Design review of the part built by this model. Coordinates are the model's own, in mm. A direction names the side the tool comes from. Round coordinates to 2 decimals unless told otherwise and drop trailing zeros. Order: outer loops, then holes, each group sorted by start corner. A loop starts at its lowest first (then second) coordinate and runs counter-clockwise, first axis right, second up. Notation, with made-up numbers: (87.5, 78.25) - (132.5, 78.25) arc R22 cw to (132.5, 94.25) - close; hole circle Ø6 at (50.25, 4.25). An arc over 180 degrees is marked (long way). Use CSV: the item, a comma, the result in double quotes. Start each with the question number.
Autodesk Inventor part; units mm, degrees
ref_plane "YZ Plane" through (0, 0, 0) normal (1, 0, 0) x (0, 1, 0)
ref_plane "XZ Plane" through (0, 0, 0) normal (0, 1, 0) x (-1, 0, 0)
ref_plane "XY Plane" through (0, 0, 0) normal (0, 0, 1) x (1, 0, 0)
sketch "Sketch1" plane through (0, 0, 0) normal (1, 0, 0) x (0, 1, 0)
  arc A0 (144.9614, 17.799) -> (0, 146.05) centre (0, 0) ccw
  line L0 (0, 0) -> (144.9614, 17.799) construction
  line L1 (0, 0) -> (0, 146.05) construction
  arc A1 (146.537, 17.9925) -> (0, 147.6375) centre (0, 0) ccw
  line L2 (0, 146.05) -> (0, 147.6375)
  line L3 (144.9614, 17.799) -> (146.537, 17.9925)
  dimension "d0" = 146.05
  dimension "d1" = 83
  dimension "d2" = 1.5875
extrude "Extrusion1" add sketch "Sketch1" along normal blind 612.775
sketch "Sketch2" plane through (612.775, 0, 0) normal (1, 0, 0) x (0, 0, -1)
  arc A0 (-17.799, 144.9614) -> (-146.05, 0) centre (0, 0) ccw construction
  line L0 (-146.05, 0) -> (0, 0) construction
  line L1 (-17.799, 144.9614) -> (0, 0) construction
  line L2 (0, 0) -> (-109.385, 96.7757) construction
  circle A1 centre (-97.8275, 86.5505) radius 3.175
  arc A2 (-17.9925, 146.537) -> (-147.6375, 0) centre (0, 0) ccw
  line L3 (-146.05, 0) -> (-17.799, 144.9614)
  line L4 (-47.9468, 139.635) -> (-87.7768, 94.6153)
  line L5 (-87.7768, 94.6153) -> (-101.7488, 106.9767)
  line L6 (-104.6074, 75.5919) -> (-118.5794, 87.9532)
  line L7 (-89.4123, 96.0622) -> (-106.2428, 77.0388) construction
  line L8 (-87.7768, 94.6153) -> (-104.6074, 75.5919) construction
  line L9 (-104.6074, 75.5919) -> (-144.4374, 30.5722)
  arc A3 (-101.7488, 106.9767) -> (-118.5794, 87.9532) centre (0, 0) ccw
  arc A4 (-144.4374, 30.5722) -> (-147.6375, 0) centre (0, 0) ccw
  line L10 (-147.6375, 0) -> (-146.05, 0)
  line L11 (-146.05, 0) -> (-147.6375, 0)
  arc A5 (-17.9925, 146.537) -> (-47.9468, 139.635) centre (0, 0) ccw
  line L12 (-17.799, 144.9614) -> (-17.9925, 146.537)
  line L13 (-17.9925, 146.537) -> (-17.799, 144.9614)
  line L14 (-54.9573, 131.7111) -> (-40.6897, 119.0882) construction
  circle A6 centre (-47.8235, 125.3997) radius 4.7625
  dimension "d5" = 6.35
  dimension "d6" = 130.6186
  dimension "d7" = 25.4
  dimension "d8" = 19.05
  dimension "d19" = 62.23
  dimension "d23" = 9.525
extrude "Extrusion2" add sketch "Sketch2" along normal blind 1.5875 contours L12 L3 L10 A2 L9 L6 L5 L4
sketch "Sketch3" plane through (0, 0, 0) normal (-1, 0, 0) x (0, 0, 1)
  arc A0 (146.05, 0) -> (142.2671, 33.0253) centre (0, 0) ccw
  line L0 (104.6074, 75.5919) -> (142.2671, 33.0253)
  line L1 (117.3859, 86.8973) -> (104.6074, 75.5919)
  arc A1 (117.3859, 86.8973) -> (100.5554, 105.9208) centre (0, 0) ccw
  line L2 (87.7768, 94.6153) -> (100.5554, 105.9208)
  line L3 (50.1171, 137.1819) -> (87.7768, 94.6153)
  arc A2 (50.1171, 137.1819) -> (17.799, 144.9614) centre (0, 0) ccw
  line L4 (146.05, 0) -> (17.799, 144.9614)
  circle A3 centre (97.8275, 86.5505) radius 3.175
  arc A4 (146.05, 0) -> (17.799, 144.9614) centre (0, 0) ccw
  line L5 (146.05, 0) -> (147.6375, 0)
  arc A5 (147.6375, 0) -> (17.9925, 146.537) centre (0, 0) ccw
  line L6 (17.9925, 146.537) -> (17.799, 144.9614)
extrude "Extrusion3" add sketch "Sketch3" along normal blind 1.5875 contours L4 A2 L3 L2 A1 L1 L0 A0 | A0 A4 A1 A2 L6 A5 L5
properties part number "Kick Plate"
Q1. For L1, parallel to X at y = 94.5, z = 70 (1 decimal); L2, parallel to Z at x = 480, y = 106; L3, parallel to Y at x = 374, z = 93, list the stretches that pass through material, from the lowest coordinate up. Write a range as [from, to].
Q2. Take a section at C-C (y = 24). State the section outline as (x, z) points (1 decimal), plus the area to 3 significant figures.
Q3. Take a section at D-D (z = 33). State the section outline as (x, y) points (1 decimal).
Q4. Take a section at B-B (y = 64.5). State the section outline as (x, z) points (1 decimal), plus the area to 3 significant figures.
Q5. Tool access review of faces 4 (the cylindrical face through (302.88, 96.7, 111.56)), 5 (the flat face through (612.775, 78, 92)): name each direction out of +Z, -Z, +X, -X, +Y, -Y from which nothing blocks a thin tool from reaching the whole face with its end or side.
Q6. Take a section at A-A (z = 73.5). State the section outline as (x, y) points (1 decimal).
Q7. The part is to be moulded in two halves that separate along Z. For faces 1 (the flat face through (-0.78, 71.47, 82.82)), 2 (the flat face through (613.56, 81.69, 111.5)), 3 (the flat face through (613.558, 100.709, 94.665)), say which applies: +Z half, -Z half, draft (parallel to the pull), parting line (faces both ways), or undercut.
Q8. Clearance check with flat-ended pins moving along their axes: pin 1 (1.5 mm diameter, centred on x = 145.5, z = 63.5, fed in from -Y); pin 2 (10 mm diameter, centred on y = 115, z = 87, fed in from +X) (3 decimals); pin 3 (2 mm diameter, centred on x = 194.5, z = 64.5, fed in from -Y). State where each tip first meets the part, or that it passes through.
Findings below:
1,L1,"x = [-1.6, 0], [612.8, 614.4]"
1,L2,"z = [100.47, 102.77]"
1,L3,"y = [112.61, 114.66]"
2,outline,"(-1.6, 124.8) - (0, 124.8) - (0, 144.1) - (612.8, 144.1) - (612.8, 124.8) - (614.4, 124.8) - (614.4, 145.7) - (-1.6, 145.7) - close"
2,area,"1,050 mm^2"
3,outline,"(-1.6, 127.8) - (0, 127.8) - (0, 142.3) - (612.8, 142.3) - (612.8, 127.8) - (614.4, 127.8) - (614.4, 143.9) - (-1.6, 143.9) - close"
4,outline,"(-1.6, 89) - (0, 89) - (0, 114.4) - (-1.6, 114.4) - close; (-1.6, 131) - (612.8, 131) - (612.8, 132.8) - (-1.6, 132.8) - close; (612.8, 89) - (614.4, 89) - (614.4, 114.4) - (612.8, 114.4) - close"
4,area,"1,170 mm^2"
5,face 4,"+Z, +X, -X, +Y"
5,face 5,"-Z, -Y"
6,outline,"(-1.6, 82) - (0, 82) - (0, 110.8) - (-1.6, 110.8) - close; (-1.6, 126.2) - (612.8, 126.2) - (612.8, 128) - (-1.6, 128) - close; (612.8, 82) - (614.4, 82) - (614.4, 110.8) - (612.8, 110.8) - close"
7,face 1,"-Z half"
7,face 2,"+Z half"
7,face 3,"undercut"
8,pin 1,"stops at y = 131.16"
8,pin 2,"stops at x = 612.775"
8,pin 3,"stops at y = 130.54"
